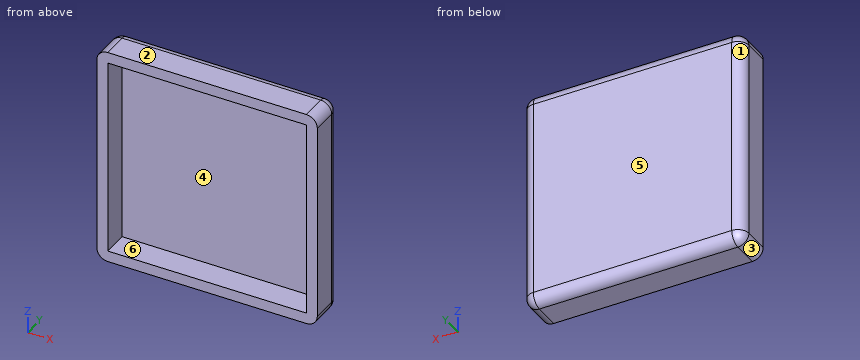
```python
from build123d import *

# Parameters (mm, degrees)
SKETCH1_W           = 1524
SKETCH1_H           = 1524
BOSS_EXTRUDE1_DEPTH = 254
FILLET1_R           = 76.2
SHELL1_START        = -685.8
SHELL1_OUTLINE_W    = 177.8
SHELL1_OUTLINE_H    = 1371.6
SHELL1_DEPTH        = 1371.6
SCALE1_SCALE        = 0.02


# Read off the part's stored shape, not the designer's step: Shell1
with BuildPart() as part:
    # Sketch1 → Boss-Extrude1 (new body)
    with BuildSketch(Plane(origin=(0, 0, 0), x_dir=(1, 0, 0), z_dir=(0, 1, 0))):
        Rectangle(SKETCH1_W, SKETCH1_H)
    extrude(amount=BOSS_EXTRUDE1_DEPTH)

    # Fillet1
    fillet1_edges = [part.edges().sort_by_distance(p)[0] for p in [
        (-762, 254, 0),
        (0, 254, 762),
        (762, 254, 0),
        (762, 127, 762),
        (-762, 127, 762),
        (-762, 127, -762),
        (762, 127, -762),
        (0, 254, -762),
    ]]
    fillet(fillet1_edges, radius=FILLET1_R)

    # Shell1 outline → Shell1 (cut)
    with BuildSketch(Plane.YZ.offset(SHELL1_START)):
        with Locations((88.9, 0)):
            Rectangle(SHELL1_OUTLINE_W, SHELL1_OUTLINE_H)
    extrude(amount=SHELL1_DEPTH, mode=Mode.SUBTRACT)


with BuildPart() as part_1:
    # Scale1: scaled about (0, 175.373677195, 0)
    add(part.part.scale(SCALE1_SCALE).moved(Location((0, 171.866203651, 0))))


solid = part_1.part
```
Could you check a few things on this model? Use its own coordinates, in mm. Face numbers are marked on the shaded views. A direction names the side the tool comes from. Round coordinates to 2 decimals unless told otherwise and drop trailing zeros. Loops run counter-clockwise (first coordinate to the right, second up) from the corner with the lowest first, then second, coordinate; pieces in that order, holes last. Notation, with made-up numbers: (26, 31.25) - (81, 31.25) arc R20 cw to (81, 35.25) - close; hole circle Ø11 at (87.25, -10.75). An arc over 180 degrees is marked (long way). Use CSV: the item, a comma, the result in double quotes.
Item 1: If we section it at A-A on y = 173.8: List the corners of the cut face in (x, z) for me.
Here are the results:
outline,"(-15.24, -13.72) arc R1.52 ccw to (-13.72, -15.24) - (13.72, -15.24) arc R1.52 ccw to (15.24, -13.72) - (15.24, 13.72) arc R1.52 ccw to (13.72, 15.24) - (-13.72, 15.24) arc R1.52 ccw to (-15.24, 13.72) - close; hole (-13.72, -13.72) - (13.72, -13.72) - (13.72, 13.72) - (-13.72, 13.72) - close"
Item 2: I need wall thicknesses on L1, parallel to X at y = 174.3, z = -5; L2, parallel to X at y = 175.5, z = 2. Which ranges of each line are inside material? Lowest first, please. Write a range as [from, to].
Here are the results:
L1,"x = [-15.24, -13.72], [13.72, 15.24]"
L2,"x = [-15.24, 15.24]"
Item 3: Will this pin go through, and if not, where does the flat tip stop? pin 1 (4 mm diameter, centred on x = 8, z = -2.5, fed in from -Y).
Here are the results:
pin 1,"stops at y = 175.42"
Item 4: For the marked faces 5 and 6, which set-ups out of +Z, -Z, +X, -X, +Y, -Y let a thin tool reach every point of the face, with its end or its side?
Here are the results:
face 5,"+Z, -Z, +X, -X, +Y"
face 6,"-Y"
Item 5: If we section it at C-C on x = 7: List the corners of the cut face in (y, z) for me, then the cut area to 3 significant figures.
Here are the results:
outline,"(171.87, -15.24) - (175.42, -15.24) arc R1.52 ccw to (176.95, -13.72) - (176.95, 13.72) arc R1.52 ccw to (175.42, 15.24) - (171.87, 15.24) - (171.87, 13.72) - (175.42, 13.72) - (175.42, -13.72) - (171.87, -13.72) - close"
area,"56.3 mm²"
Item 6: If we section it at B-B on z = 11: List the corners of the cut face in (x, y) for me, then the cut area to 3 significant figures.
Here are the results:
outline,"(-15.24, 171.87) - (-13.72, 171.87) - (-13.72, 175.42) - (13.72, 175.42) - (13.72, 171.87) - (15.24, 171.87) - (15.24, 175.42) arc R1.52 ccw to (13.72, 176.95) - (-13.72, 176.95) arc R1.52 ccw to (-15.24, 175.42) - close"
area,"56.3 mm²"
Item 7: If we mould it in two halves opening along Z, with no side actions, what happens to the marked faces 1, 2, 3 and 4? For each: pulls with the +Z half, pulls with the -Z half, needs draft (parallel to the pull), parting line crosses it, or undercut.
Here are the results:
face 1,"needs draft"
face 2,"pulls with the +Z half"
face 3,"pulls with the -Z half"
face 4,"undercut"
